Source: CAD feature listing. Evaluate the final solid. Frame: model axes, mm. A direction names the side the tool comes from. Coordinates: 2 decimals unless noted, no trailing zeros. Loops run counter-clockwise (first coordinate to the right, second up) from the corner with the lowest first, then second, coordinate; pieces in that order, holes last. Notation, with made-up numbers: (48, 45) -> (107, 45) arc R22 ccw to (107, 61) -> close; hole circle Ø11 at (3.25, 32.5). An arc over 180 degrees is marked (long way). Answer as CSV lines item,"result".
from build123d import *

# Parameters (mm, degrees)
SKETCH1_R           = 7.5
BOSS_EXTRUDE1_DEPTH = 10
BOSS_EXTRUDE2_DEPTH = 50
SKETCH3_R           = 15
CUT_EXTRUDE1_DEPTH  = 10
CUT_EXTRUDE2_START  = -30
CUT_EXTRUDE2_DEPTH  = 30
SKETCH6_W           = 25
SKETCH6_H           = 30
CUT_EXTRUDE3_DEPTH  = 30
SKETCH7_R           = 5
CUT_EXTRUDE4_DEPTH  = 30
SKETCH8_R           = 5.1
CUT_EXTRUDE5_DEPTH  = 5
SKETCH9_R           = 1.5
CUT_EXTRUDE6_DEPTH  = 71
CIRPATTERN1_COUNT   = 2
CIRPATTERN1_ANGLE   = 90


with BuildPart() as part:
    # Sketch1 → Boss-Extrude1 (new body)
    with BuildSketch(Plane.XY):
        Circle(SKETCH1_R)
    extrude(amount=BOSS_EXTRUDE1_DEPTH)

    # Sketch2 → Boss-Extrude2 (add)
    with BuildSketch(Plane.XY.offset(10)):
        with BuildLine():
            Line((20, 0), (20, 30))
            Line((20, 30), (-20, 30))
            Line((-20, 30), (-20, 0))
            ThreePointArc((-20, 0), (0, -20), (20, 0))
        make_face()
    extrude(amount=BOSS_EXTRUDE2_DEPTH)

    # Sketch3 → Cut-Extrude1 (cut)
    with BuildSketch(Plane.XY.offset(60)):
        Circle(SKETCH3_R)
    extrude(amount=-CUT_EXTRUDE1_DEPTH, mode=Mode.SUBTRACT)

    # Sketch5 → Cut-Extrude2 (cut)
    with BuildSketch(Plane(origin=(0, 0, 15), x_dir=(-1, 0, 0), z_dir=(0, 0, -1)).offset(CUT_EXTRUDE2_START)):
        with BuildLine():
            Line((15, 25), (-15, 25))
            Line((-15, 25), (-15, 0))
            ThreePointArc((-15, 0), (0, -15), (15, 0))
            Line((15, 0), (15, 25))
        make_face()
    extrude(amount=CUT_EXTRUDE2_DEPTH, mode=Mode.SUBTRACT)

    # Sketch6 → Cut-Extrude3 (cut)
    with BuildSketch(Plane(origin=(0, 30, 0), x_dir=(1, 0, 0), z_dir=(0, 1, 0))):
        with Locations((0, -30)):
            Rectangle(SKETCH6_W, SKETCH6_H)
    extrude(amount=-CUT_EXTRUDE3_DEPTH, mode=Mode.SUBTRACT)

    # Sketch7 → Cut-Extrude4 (cut)
    with BuildSketch(Plane.XY.offset(50)):
        Circle(SKETCH7_R)
    extrude(amount=-CUT_EXTRUDE4_DEPTH, mode=Mode.SUBTRACT)

    # Sketch8 → Cut-Extrude5 (cut)
    with BuildSketch(Plane(origin=(0, 0, 0), x_dir=(-1, 0, 0), z_dir=(0, 0, -1))):
        Circle(SKETCH8_R)
    extrude(amount=-CUT_EXTRUDE5_DEPTH, mode=Mode.SUBTRACT)

    # Sketch9 → Cut-Extrude6 (cut, symmetric)
    with BuildSketch(Plane(origin=(0, 0, 0), x_dir=(1, 0, 0), z_dir=(0, 1, 0))):
        with Locations(Location((0, -2.5, 0), (0, 0, 270))):
            Circle(SKETCH9_R)
    cut_extrude6 = extrude(amount=CUT_EXTRUDE6_DEPTH, both=True, mode=Mode.SUBTRACT)

    # CirPattern1: Cut-Extrude6 ×2 about axis
    cirpattern1_axis = Axis((0, 0, 0), (0, 0, 1))
    for i in range(1, CIRPATTERN1_COUNT):
        add(cut_extrude6.rotate(cirpattern1_axis, i * CIRPATTERN1_ANGLE / (CIRPATTERN1_COUNT - 1)), mode=Mode.SUBTRACT)


solid = part.part
(1) Material intervals for L1, parallel to Z at x = 6.1, y = 0; L2, parallel to Z at x = 6.5, y = -9.5; L3, parallel to X at y = 13.5, z = 21, sorted ascending. Write a range as [from, to].
Computed values:
L1,"[0, 1], [4, 15], [45, 50]"
L2,"[10, 15], [45, 50]"
L3,"[-20, -15], [15, 20]"
(2) Cut plane A-A (x = 0). State how many separate pieces and enclosed holes the cut face has, then the cut area to 3 significant figures.
Computed values:
separate pieces,"4"
enclosed holes,"0"
area,"885 mm^2"
(3) Draft query along Z for faces 1 (the flat face through (0, 16, 60)), 2 (the cylindrical face through (-1.08, -4.88, 47.54)), 3 (the flat face through (14, 25, 30)). Return one class per face: released by +Z, released by -Z, zero draft, split by the parting line, or undercut.
Computed values:
face 1,"released by +Z"
face 2,"zero draft"
face 3,"undercut"
(4) Pin query (flat end, axial travel): pin 1 Ø3 at (x, z) = (14.5, 26.5) entering from -Y; pin 2 Ø8 at (x, y) = (0, 0) entering from +Z; pin 3 Ø9 at (x, y) = (3, 4.5) entering from +Z. Return the tip coordinate at first contact, or that it passes through.
Computed values:
pin 1,"y = -15.2"
pin 2,"z = 15"
pin 3,"z = 50"
(5) Access query for faces 4 (the flat face through (0, 8, 45)), 5 (the flat face through (-4, 4, 50)), 6 (the cylindrical face through (0, -20, 35)), 7 (the flat face through (-12.5, 28, 30)), 8 (the flat face through (0, 0, 5)). Directions: +Z, -Z, +X, -X, +Y, -Y. A direction counts if a zero-diameter tool reaches every point of the face in a straight line with its end or side. Return the directions, or none.
Computed values:
face 4,"none"
face 5,"+Z"
face 6,"+Z, -Z, -Y"
face 7,"+Y"
face 8,"-Z"
(6) Cut plane D-D (z = 48). Return the cut outline in (x, y), then the cut area to 3 significant figures.
Computed values:
outline,"(-20, 0) arc R20 ccw to (20, 0) -> (20, 30) -> (-20, 30) -> close; hole circle Ø10 at (0, 0)"
area,"1,750 mm^2"
(7) Cut plane C-C (z = 2.5). Return the cut outline in (x, y).
Computed values:
outline,"(-7.35, -1.5) arc R7.5 ccw to (-1.5, -7.35) -> (-1.5, -4.87) arc R5.1 cw to (-4.87, -1.5) -> close; (-7.35, 1.5) -> (-4.87, 1.5) arc R5.1 cw to (-1.5, 4.87) -> (-1.5, 7.35) arc R7.5 ccw to start; (1.5, -7.35) arc R7.5 ccw to (7.35, -1.5) -> (4.87, -1.5) arc R5.1 cw to (1.5, -4.87) -> close; (1.5, 4.87) arc R5.1 cw to (4.87, 1.5) -> (7.35, 1.5) arc R7.5 ccw to (1.5, 7.35) -> close"
(8) Cut plane B-B (y = 23). Return the cut outline in (x, z), then the cut area to 3 significant figures.
Computed values:
outline,"(-20, 10) -> (20, 10) -> (20, 60) -> (-20, 60) -> close; hole (-15, 15) -> (15, 15) -> (15, 45) -> (-15, 45) -> close"
area,"1,100 mm^2"
